```python
from build123d import *

# Parameters (mm, degrees)
F0_R     = 17.5
F1_DEPTH = 25
F2_R     = 5
F3_SIZE  = 1
F4_D     = 6.5278
F4_DEPTH = 16.2333333333
F4_TIP   = 1.9611489744


with BuildPart() as f1:
    # F0 (on Top) → F1 (new body)
    with BuildSketch(Plane.XY):
        Circle(F0_R)
    extrude(amount=F1_DEPTH)

    # F2
    f2_edges = [f1.edges().sort_by_distance(p)[0] for p in [
        (-17.5, 0, 25),
    ]]
    fillet(f2_edges, radius=F2_R)

    # F3
    f3_edges = [f1.edges().sort_by_distance(p)[0] for p in [
        (-17.5, 0, 0),
    ]]
    chamfer(f3_edges, length=F3_SIZE)

    # F4
    with Locations(Plane(origin=(0, 0, 0), x_dir=(1, 0, 0), z_dir=(0, 0, -1))):
        with Locations((0, 0)):
            Hole(F4_D / 2, depth=F4_DEPTH)
            with Locations((0, 0, -(F4_DEPTH + F4_TIP / 2))):  # 118° drill point
                Cone(0, F4_D / 2, F4_TIP, mode=Mode.SUBTRACT)


solid = f1.part
```
Input: part model. Units: mm. Frame: model coordinates. Round coordinates to 2 decimals unless told otherwise and drop trailing zeros. Loops run counter-clockwise (first coordinate to the right, second up) from the corner with the lowest first, then second, coordinate; pieces in that order, holes last. Notation, with made-up numbers: M 47,73.5 L 92,73.5 A14 cw 92,88.5 Z; hole C -12,41 d5. An arc over 180 degrees is marked long. Answer in a Markdown table with one row per item. Add a question column.
1. Ray query, probe 1 along Y at (x, z) = (0, 3.75); probe 2 along Y at (x, z) = (2, 6.75); probe 3 along Z at (x, y) = (14, -5). Return the intervals inside material, ascending.
2. Section B-B (z = 22). Output: boundary loops of the cut face in (x, y), and give its area (3 significant figures).
3. Section A-A (z = 3). Output: boundary loops of the cut face in (x, y), and give its area (3 significant figures).
4. Contact query for flat-ended pins moving along their axis: pin 1 (3 mm diameter, centred on x = 9.5, z = 21.5, fed in from -Y); pin 2 (2 mm diameter, centred on x = 9, z = 11.5, fed in from -Y); pin 3 (5 mm diameter, centred on x = -8.5, z = 14.5, fed in from -Y). Output: stop coordinate, or through.
5. Mould query, pull axis X, two halves, no side actions, for faces 1 (the face through (0.708, 3.186, 8.23)), 2 (the face through (0.541, -0.17, 17.854)), 3 (the face through (-13.887, -10.648, 10.367)), 4 (the face through (0, 0, 25)). Classes: released by +X, released by -X, zero draft, split by the parting line, or undercut.
Values follow:
| question | item | result |
|---|---|---|
| 1 | probe 1 | -17.5 to -3.26, 3.26 to 17.5 |
| 1 | probe 2 | -17.39 to -2.58, 2.58 to 17.39 |
| 1 | probe 3 | 0 to 24.4 |
| 2 | outline | C 0,0 d34.17 |
| 2 | area | 917 mm^2 |
| 3 | outline | C 0,0 d35; hole C 0,0 d6.53 |
| 3 | area | 929 mm^2 |
| 4 | pin 1 | y = -15.41 |
| 4 | pin 2 | y = -15.56 |
| 4 | pin 3 | y = -16.44 |
| 5 | face 1 | undercut |
| 5 | face 2 | undercut |
| 5 | face 3 | split by the parting line |
| 5 | face 4 | zero draft |
